```python
from build123d import *

# Parameters (mm, degrees)
BOSS_EXTRUDE1_DEPTH = 1.5
SKETCH2_R           = 1.5
CUT_EXTRUDE1_DEPTH  = 108.510464607
FILLET1_R           = 7
SKETCH3_R           = 1.5
CUT_EXTRUDE2_DEPTH  = 105.519616835
SKETCH6_R           = 1.25
CUT_EXTRUDE3_DEPTH  = 105.519616835
SKETCH8_W           = 25
SKETCH8_H           = 2
BOSS_EXTRUDE2_DEPTH = 1.5


with BuildPart() as part:
    # Sketch1 → Boss-Extrude1 (new body)
    with BuildSketch(Plane(origin=(0, 0, 0), x_dir=(1, 0, 0), z_dir=(0, 1, 0))):
        with BuildLine():
            Line((76.013978978, 8.838834765), (58.336309448, -8.838834765))
            ThreePointArc((58.336309448, -8.838834765), (33.587572106, 0), (8.838834765, -8.838834765))
            Line((8.838834765, -8.838834765), (-8.838834765, 8.838834765))
            ThreePointArc((-8.838834765, 8.838834765), (0, 33.587572106), (-8.838834765, 58.336309448))
            Line((-8.838834765, 58.336309448), (8.838834765, 76.013978978))
            ThreePointArc((8.838834765, 76.013978978), (33.587572106, 67.175144213), (58.336309448, 76.013978978))
            Line((58.336309448, 76.013978978), (76.013978978, 58.336309448))
            ThreePointArc((76.013978978, 58.336309448), (67.175144213, 33.587572106), (76.013978978, 8.838834765))
        make_face()
    extrude(amount=BOSS_EXTRUDE1_DEPTH)

    # Sketch2 → Cut-Extrude1 (cut, through all)
    with BuildSketch(Plane(origin=(0, 1.5, 0), x_dir=(1, 0, 0), z_dir=(0, 1, 0))):
        with Locations(Location((57.629202667, 68.235804385, 0), (0, 0, 270))):
            Circle(SKETCH2_R)
        with Locations(Location((68.235804385, 57.629202667, 0), (0, 0, 270))):
            Circle(SKETCH2_R)
        with Locations(Location((68.235804385, 9.545941546, 0), (0, 0, 270))):
            Circle(SKETCH2_R)
        with Locations(Location((57.629202667, -1.060660172, 0), (0, 0, 270))):
            Circle(SKETCH2_R)
        with Locations(Location((9.545941546, -1.060660172, 0), (0, 0, 270))):
            Circle(SKETCH2_R)
        with Locations(Location((-1.060660172, 9.545941546, 0), (0, 0, 270))):
            Circle(SKETCH2_R)
        with Locations(Location((-1.060660172, 57.629202667, 0), (0, 0, 270))):
            Circle(SKETCH2_R)
        with Locations(Location((9.545941546, 68.235804385, 0), (0, 0, 270))):
            Circle(SKETCH2_R)
    extrude(amount=-CUT_EXTRUDE1_DEPTH, mode=Mode.SUBTRACT)

    # Fillet1
    fillet1_edges = [part.edges().sort_by_distance(p)[0] for p in [
        (76.013978978, 0.75, -8.838834765),
        (58.336309448, 0.75, 8.838834765),
        (8.838834765, 0.75, 8.838834765),
        (-8.838834765, 0.75, -8.838834765),
        (-8.838834765, 0.75, -58.336309448),
        (8.838834765, 0.75, -76.013978978),
        (58.336309448, 0.75, -76.013978978),
        (76.013978978, 0.75, -58.336309448),
    ]]
    fillet(fillet1_edges, radius=FILLET1_R)

    # Sketch3 → Cut-Extrude2 (cut, through all)
    with BuildSketch(Plane(origin=(0, 1.5, 0), x_dir=(1, 0, 0), z_dir=(0, 1, 0))):
        with Locations(Location((18.087572106, 49.087572106, 0), (0, 0, 270))):
            Circle(SKETCH3_R)
        with Locations(Location((18.087572106, 18.087572106, 0), (0, 0, 270))):
            Circle(SKETCH3_R)
        with Locations(Location((49.087572106, 18.087572106, 0), (0, 0, 90))):
            Circle(SKETCH3_R)
        with Locations(Location((49.087572106, 49.087572106, 0), (0, 0, 90))):
            Circle(SKETCH3_R)
    extrude(amount=-CUT_EXTRUDE2_DEPTH, mode=Mode.SUBTRACT)

    # Sketch6 → Cut-Extrude3 (cut, through all)
    with BuildSketch(Plane(origin=(0, 1.5, 0), x_dir=(1, 0, 0), z_dir=(0, 1, 0))):
        with Locations(Location((58.587572106, 46.087572106, 0), (0, 0, 270))):
            Circle(SKETCH6_R)
        with Locations(Location((58.587572106, 21.087572106, 0), (0, 0, 270))):
            Circle(SKETCH6_R)
        with Locations(Location((8.587572106, 21.087572106, 0), (0, 0, 90))):
            Circle(SKETCH6_R)
        with Locations(Location((8.587572106, 46.087572106, 0), (0, 0, 90))):
            Circle(SKETCH6_R)
        with BuildLine():
            Line((23.587572106, 58.087572106), (43.587572106, 58.087572106))
            ThreePointArc((43.587572106, 58.087572106), (45.087572106, 56.587572106), (43.587572106, 55.087572106))
            Line((43.587572106, 55.087572106), (23.587572106, 55.087572106))
            ThreePointArc((23.587572106, 55.087572106), (22.087572106, 56.587572106), (23.587572106, 58.087572106))
        make_face()
        with BuildLine():
            Line((23.587572106, 9.087572106), (43.587572106, 9.087572106))
            ThreePointArc((43.587572106, 9.087572106), (45.087572106, 10.587572106), (43.587572106, 12.087572106))
            Line((43.587572106, 12.087572106), (23.587572106, 12.087572106))
            ThreePointArc((23.587572106, 12.087572106), (22.087572106, 10.587572106), (23.587572106, 9.087572106))
        make_face()
        Polygon((33.587572106, 48.021328836), (21.087572106, 40.804450471), (21.087572106, 26.370693741), (33.587572106, 19.153815377), (46.087572106, 26.370693741), (46.087572106, 40.804450471), align=None)
    extrude(amount=-CUT_EXTRUDE3_DEPTH, mode=Mode.SUBTRACT)

    # Sketch8 → Boss-Extrude2 (add, through all)
    with BuildSketch(Plane(origin=(0, 1.5, 0), x_dir=(1, 0, 0), z_dir=(0, 1, 0))):
        with Locations((33.587572106, 35.587572106)):
            Rectangle(SKETCH8_W, SKETCH8_H)
        with Locations((33.587572106, 31.587572106)):
            Rectangle(SKETCH8_W, SKETCH8_H)
        with Locations((33.587572106, 39.587572106)):
            Rectangle(SKETCH8_W, SKETCH8_H)
        Polygon((24.176029374, 42.587572106), (42.999114838, 42.587572106), (39.535013223, 44.587572106), (27.64013099, 44.587572106), align=None)
        with Locations((33.587572106, 27.587572106)):
            Rectangle(SKETCH8_W, SKETCH8_H)
        Polygon((39.535013223, 22.587572106), (42.999114838, 24.587572106), (24.176029374, 24.587572106), (27.64013099, 22.587572106), align=None)
    extrude(amount=-BOSS_EXTRUDE2_DEPTH)


solid = part.part
```
Source: CAD feature listing. Evaluate the final solid. Frame: model axes, mm. A direction names the side the tool comes from. Round coordinates to 2 decimals unless told otherwise and drop trailing zeros. Loops run counter-clockwise (first coordinate to the right, second up) from the corner with the lowest first, then second, coordinate; pieces in that order, holes last. Notation, with made-up numbers: M 82,-11 L 124,-11 A24 cw 124,4 Z; hole C 71,87 d11. An arc over 180 degrees is marked long. Use a Markdown table: item, result. Add a question column.
1. Line query: line 1 (Z direction, x = 57, y = 0.25); line 2 (Z direction, x = 19, y = 0.25); line 3 (X direction, y = 0.3, z = -20.5). Output: solid intervals per line, ascending.
2. Section query D-D on z = -64. Return the cut outline in (x, y), then the cut area to 3 significant figures.
3. Mould query, pull axis Z, two halves, no side actions, for faces 1 (the cylindrical face through (58.45, 0.76, -73.84)), 2 (the cylindrical face through (58.449, 0.76, 6.666)), 3 (the cylindrical face through (58.109, 0.76, -19.933)). Classes: pulls with the +Z half, pulls with the -Z half, needs draft (parallel to the pull), parting line crosses it, or undercut.
4. Section query C-C on y = 0.4. Give the number of separate pieces and of enclosed holes in the cut face, then the cut area to 3 significant figures.
5. Section query B-B on x = 2. Return the cut outline in (y, z).
6. Reachability of faces 4 (the flat face through (44.522, 0.76, -25.467)), 5 (the flat face through (67.11, 0.74, -67.24)) from +Z, -Z, +X, -X, +Y, -Y: full face, straight path, thin tool, end or side. Return the list, or none.
7. Section query A-A on z = -10. Return the cut outline in (x, y).
Reported:
| question | item | result |
|---|---|---|
| 1 | line 1 | z = -73.88 to -69.6, -66.87 to -0.3, 2.42 to 6.7 |
| 1 | line 2 | z = -70 to -50.28, -47.9 to -19.28, -16.9 to 2.83 |
| 1 | line 3 | x = -2.26 to 7.48, 9.69 to 31.26, 35.92 to 57.48, 59.69 to 69.43 |
| 2 | outline | M -3.18,0 L 70.35,0 L 70.35,1.5 L -3.18,1.5 Z |
| 2 | area | 110 mm² |
| 3 | face 1 | pulls with the -Z half |
| 3 | face 2 | pulls with the +Z half |
| 3 | face 3 | undercut |
| 4 | separate pieces | 1 |
| 4 | enclosed holes | 25 |
| 4 | area | 4,810 mm² |
| 5 | outline | M 0,-69.18 L 1.5,-69.18 L 1.5,2 L 0,2 Z |
| 6 | face 4 | +Y, -Y |
| 6 | face 5 | -Z, +X, +Y, -Y |
| 7 | outline | M -6.71,0 L -2.49,0 L -2.49,1.5 L -6.71,1.5 Z; M 0.37,0 L 22.21,0 L 22.21,1.5 L 0.37,1.5 Z; M 44.97,0 L 66.81,0 L 66.81,1.5 L 44.97,1.5 Z; M 69.67,0 L 73.89,0 L 73.89,1.5 L 69.67,1.5 Z |
